Check sheet for the modelled part. Datum: model origin and axes. Units: mm. A direction names the side the tool comes from. Give positions to 0.01 mm unless a question says otherwise; leave off trailing zeros. Loops run counter-clockwise (first coordinate to the right, second up) from the corner with the lowest first, then second, coordinate; pieces in that order, holes last. Notation, with made-up numbers: (38.5, -17) - (70.5, -17) arc R23 ccw to (70.5, -4) - close; hole circle Ø9 at (30, 82.25). An arc over 180 degrees is marked (long way). Use one line per item in the form item = value.
Autodesk Inventor part; units mm, degrees
ref_plane "YZ Plane" through (0, 0, 0) normal (1, 0, 0) x (0, 1, 0)
ref_plane "XZ Plane" through (0, 0, 0) normal (0, 1, 0) x (-1, 0, 0)
ref_plane "XY Plane" through (0, 0, 0) normal (0, 0, 1) x (1, 0, 0)
sketch "Sketch1" plane through (0, 0, 0) normal (0, 1, 0) x (-1, 0, 0)
  line L0 (-1, -15.5) -> (1, -15.5)
  line L1 (1, 15.5) -> (-1, 15.5)
  line L2 (-3, 13.5) -> (-3, -13.5)
  line L3 (-3, -15.5) -> (3, 15.5) construction
  line L4 (3, -15.5) -> (-3, 15.5) construction
  circle A0 centre (0, 12.5) radius 1.525
  circle A1 centre (0, -12.5) radius 1.525
  arc A2 (-1, 15.5) -> (-3, 13.5) centre (-1, 13.5) ccw
  arc A3 (-3, -13.5) -> (-1, -15.5) centre (-1, -13.5) ccw
  line L5 (1, -15.5) -> (9, -15.5)
  line L6 (11, -13.5) -> (11, 13.5)
  line L7 (9, 15.5) -> (1, 15.5)
  arc A4 (9, -15.5) -> (11, -13.5) centre (9, -13.5) ccw
  arc A5 (11, 13.5) -> (9, 15.5) centre (9, 13.5) ccw
  point P0 (0, 0)
  point P1 (11, -15.5)
  dimension "d0" = 25
  dimension "d1" = 3.05
  dimension "d2" = 3.05
  dimension "d3" = 3
  dimension "d4" = 3
  dimension "d7" = 31
  dimension "d19" = 10
  dimension "d20" = 2
extrude "Extrusion1" add sketch "Sketch1" along normal blind 5
sketch "Sketch2" plane through (3, 0, 13.5) normal (1, 0, 0) x (0, 0, -1)
  line L0 (0, 5) -> (27, 5)
  line L1 (27, 5) -> (0, 5)
  line L2 (13.5, 5) -> (13.5, 10)
  line L3 (13.5, 10) -> (17.7859, 10)
  line L4 (18.2558, 9.329) -> (16.6801, 5)
  line L5 (13.5, 10) -> (9.2141, 10)
  line L6 (8.7442, 9.329) -> (10.3199, 5)
  line L7 (10.3199, 5) -> (16.6801, 5)
  arc A0 (9.2141, 10) -> (8.7442, 9.329) centre (9.2141, 9.5) ccw
  arc A1 (18.2558, 9.329) -> (17.7859, 10) centre (17.7859, 9.5) ccw
  point P0 (13.5, 0)
  point P1 (18.5, 10)
  point P2 (8.5, 10)
  dimension "d11" = 5
  dimension "d12" = 5
  dimension "d13" = 70
  dimension "d14" = 5
  dimension "d15" = 70
  dimension "d16" = 0.5
extrude "Extrusion2" add sketch "Sketch2" against normal up to surface (14 mm away)
sketch "Sketch3" plane through (3, 10, 4.2859) normal (0, 1, 0) x (1, 0, 0)
  line L0 (-14, 8.5719) -> (-14, 0)
  line L1 (-14, 1.7859) -> (-19, 1.7859)
  line L2 (-19, 1.7859) -> (-19, 6.7859)
  line L3 (-19, 6.7859) -> (-14, 6.7859)
  line L4 (-14, 6.7859) -> (-14, 1.7859)
  line L5 (0, 8.5719) -> (-14, 8.5719)
  point P0 (-3, 4.2859)
  point P1 (-14, 4.2859)
  point P2 (-14, 6.7859)
  dimension "d21" = 5
  dimension "d22" = 5
extrude "Extrusion3" add sketch "Sketch3" against normal blind 1.5
sketch "Sketch4" plane through (-11, 10, -2.5) normal (0, 0, -1) x (-1, 0, 0)
  line L0 (5, 0) -> (0, 0)
  line L1 (5, 0) -> (4, 0)
  line L2 (4, 0) -> (4, 0.3382)
  line L3 (4.1447, 0.4276) -> (5, 0)
  arc A0 (4.1447, 0.4276) -> (4, 0.3382) centre (4.1, 0.3382) ccw
  point P0 (-11, -10)
  point P1 (4, 0.5)
  dimension "d26" = 1
  dimension "d27" = 0.5
  dimension "d28" = 0.1
extrude "Extrusion4" add sketch "Sketch4" against normal up to surface (5 mm away)
fillet "Fillet1" radius 2 1 edges at (-11, 8.5, 0)
fillet "Fillet2" radius 0.2 1 edges at (-16, 10, 0)
sketch "Sketch5" plane through (3, 0, 13.5) normal (1, 0, 0) x (0, 0, -1)
  line L0 (0, 0) -> (27, 0)
  line L1 (27, 0) -> (27, 5)
  line L2 (16.6801, 5) -> (27, 5)
  line L3 (16.6801, 5) -> (18.2558, 9.329)
  arc A0 (18.2558, 9.329) -> (17.7859, 10) centre (17.7859, 9.5) ccw
  line L4 (17.7859, 10) -> (9.2141, 10)
  arc A1 (9.2141, 10) -> (8.7442, 9.329) centre (9.2141, 9.5) ccw
  line L5 (8.7442, 9.329) -> (10.3199, 5)
  line L6 (0, 5) -> (10.3199, 5)
  line L7 (0, 0) -> (0, 5)
  line L8 (9.2141, 11) -> (17.7859, 11)
  arc A2 (19.2859, 9.5) -> (17.7859, 11) centre (17.7859, 9.5) ccw
  arc A3 (9.2141, 11) -> (7.7141, 9.5) centre (9.2141, 9.5) ccw
  line L9 (7.7141, 9.5) -> (7.7141, 5)
  line L10 (19.2859, 9.5) -> (19.2859, 5)
  line L11 (7.7141, 5) -> (19.2859, 5)
  point P0 (13.5, 0)
  dimension "d33" = 1
extrude "Extrusion5" add sketch "Sketch5" against normal blind 1 contours L9 A3 L8 A2 L10 L2 L3 A0 L4 A1 L5 L6
fillet "Fillet3" radius 0.5 1 edges at (2.5, 5, 5.7859)
fillet "Fillet4" radius 0.5 3 edges at (2.5, 5, -5.7859) (-11, 8.25, 2.5) (-11, 8.25, -2.5)
equation "\"d2\" = d1"
equation "\"d4\" = d3"
properties part number "male1"
Item 1: Access from +Z, -Z, +X, -X, +Y, -Y to the whole of each face (thin tool, end or side, straight path). Record for faces 4 (the face through (-14, 9, 2.5)), 5 (the face through (-4.409, 7.195, -3.979)), 6 (the face through (2.5, 7.5, 5.786)).
Answer block:
face_4 = +Z, -X, +Y, -Y
face_5 = -Z, -X
face_6 = +Z, +X, -X, +Y
Item 2: Mould release check, pull along X, two halves, no side actions. Record for faces 1 (the face through (-11.57, 7.9, 0.04)), 2 (the face through (-6, 10, 0)), 3 (the face through (-4, 5, 9)): released by +X, released by -X, zero draft, split by the parting line, or undercut.
Answer block:
face_1 = released by -X
face_2 = undercut
face_3 = zero draft
Item 3: Section check D-D on x = -7.5. Record the boundary of the cut face in (y, z), then the cut area to 3 significant figures.
Answer block:
outline = (0, -15.5) - (5, -15.5) - (5, -3.18) - (9.33, -4.76) arc R0.5 ccw to (10, -4.29) - (10, 4.29) arc R0.5 ccw to (9.33, 4.76) - (5, 3.18) - (5, 15.5) - (0, 15.5) - close
area = 196 mm2
Item 4: Thickness scan on L1, parallel to Z at x = 0, y = 2 (3 decimals); L2, parallel to Z at x = -1, y = 4; L3, parallel to Y at x = 2, z = 12. Record the ranges inside material, lowest first.
Answer block:
L1 = -15.5 to -14.025, -10.975 to 10.975, 14.025 to 15.5
L2 = -15.5 to -13.65, -11.35 to 11.35, 13.65 to 15.5
L3 = 0 to 5
Item 5: Section check C-C on y = 4.5. Record the boundary of the cut face in (x, z) (3 decimals).
Answer block:
outline = (-11, -13.5) arc R2 ccw to (-9, -15.5) - (1, -15.5) arc R2 ccw to (3, -13.5) - (3, 13.5) arc R2 ccw to (1, 15.5) - (-9, 15.5) arc R2 ccw to (-11, 13.5) - close; hole circle Ø3.05 at (0, -12.5); hole circle Ø3.05 at (0, 12.5)
Item 6: Section check B-B on x = 0. Record the boundary of the cut face in (y, z) (3 decimals).
Answer block:
outline = (0, -15.5) - (5, -15.5) - (5, -14.025) - (0, -14.025) - close; (0, -10.975) - (5, -10.975) - (5, -3.18) - (9.329, -4.756) arc R0.5 ccw to (10, -4.286) - (10, 4.286) arc R0.5 ccw to (9.329, 4.756) - (5, 3.18) - (5, 10.975) - (0, 10.975) - close; (0, 14.025) - (5, 14.025) - (5, 15.5) - (0, 15.5) - close
Item 7: Section check A-A on z = -12.5. Record the boundary of the cut face in (x, y) (3 decimals), then the cut area to 4 significant figures.
Answer block:
outline = (-11, 0) - (-1.525, 0) - (-1.525, 5) - (-11, 5) - close; (1.525, 0) - (3, 0) - (3, 5) - (1.525, 5) - close
area = 54.75 mm2
Item 8: Gauge pin test, flat ends, axial feed: P1, Ø0.5, axis at x = 2.5, y = 7, coming from the -Z side; P2, Ø10, axis at x = -3, z = -12.5, coming from the +Y side; P3, Ø4, axis at y = 5, z = -9, coming from the -X side. Record the tip position at first contact, or that the pin passes through.
Answer block:
P1 = -5.79
P2 = 5
P3 = -11
